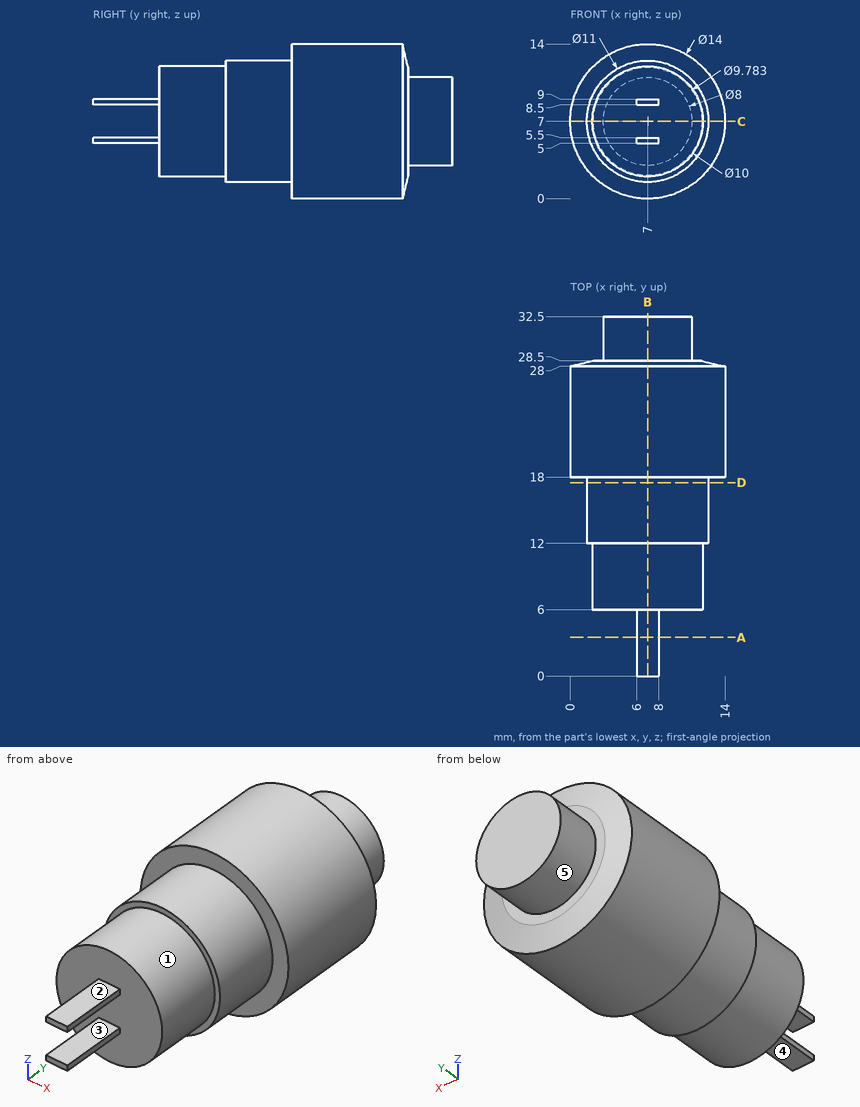
Could you check a few things on this drawing? It's one solid part, dimensions in mm from its lowest x, y, z. A direction names the side the tool comes from. Give positions to 0.01 mm unless a question says otherwise; leave off trailing zeros. Order: outer loops, then holes, each group sorted by start corner. A loop starts at its lowest first (then second) coordinate and runs counter-clockwise, first axis right, second up. Notation, with made-up numbers: (29.25, 40.5) -> (63.25, 40.5) arc R10 cw to (63.25, 52.5) -> close; hole circle Ø2 at (1, 65). An arc over 180 degrees is marked (long way). Use CSV: the item, a comma, the result in double quotes. Start each with the question number.
Item 1: On a 3-axis mill with a long thin cutter (end or side, diameter ignored), from which of +Z, -Z, +X, -X, +Y, -Y can I reach the whole of each face in a straight line? I mean the marked faces 1, 2, 3, 4 and 5. Say none if no direction works.
Item 2: Suppose I cut it at C-C (z = 7). List the corners of the cut face in (x, y) for me, and give its area (3 significant figures).
Item 3: Suppose I cut it at B-B (x = 7). List the corners of the cut face in (y, z) for me.
Item 4: Suppose I cut it at A-A (y = 3.5). List the corners of the cut face in (x, z) for me.
Item 5: I'm going to push flat-ended pins straight in: P1, Ø0.6, axis at y = 4, z = 5, coming from the +X side; P2, Ø1.5, axis at x = 5.5, y = 8, coming from the -Z side; P3, Ø5, axis at x = 4.5, z = 5.5, coming from the -Y side; P4, Ø1, axis at y = 20.5, z = 5, coming from the +X side. Where does each tip first touch, or does it pass through?
Item 6: Suppose I cut it at D-D (y = 17.5). List the corners of the cut face in (x, z) for me.
Item 7: If I drill on probe 1 along Y at (x, z) = (4, 9); probe 2 along Y at (x, z) = (3.5, 9); probe 3 along Z at (x, y) = (5.5, 31), over which ranges is the centre line in solid material (lowest first)? Write a range as [from, to].
Answer block:
1,face 1,"-Y"
1,face 2,"+Z, +X, -X, -Y"
1,face 3,"+X, -X, -Y"
1,face 4,"-Z, +X, -X, -Y"
1,face 5,"+Y"
2,outline,"(0, 18) -> (1.5, 18) -> (1.5, 12) -> (2, 12) -> (2, 6) -> (12, 6) -> (12, 12) -> (12.5, 12) -> (12.5, 18) -> (14, 18) -> (14, 28) -> (11.89, 28.5) -> (11, 28.5) -> (11, 32.5) -> (3, 32.5) -> (3, 28.5) -> (2.11, 28.5) -> (0, 28) -> close"
2,area,"304 mm^2"
3,outline,"(0, 5) -> (6, 5) -> (6, 2) -> (12, 2) -> (12, 1.5) -> (18, 1.5) -> (18, 0) -> (28, 0) -> (28.5, 2.11) -> (28.5, 3) -> (32.5, 3) -> (32.5, 11) -> (28.5, 11) -> (28.5, 11.89) -> (28, 14) -> (18, 14) -> (18, 12.5) -> (12, 12.5) -> (12, 12) -> (6, 12) -> (6, 9) -> (0, 9) -> (0, 8.5) -> (6, 8.5) -> (6, 5.5) -> (0, 5.5) -> close"
4,outline,"(6, 5) -> (8, 5) -> (8, 5.5) -> (6, 5.5) -> close; (6, 8.5) -> (8, 8.5) -> (8, 9) -> (6, 9) -> close"
5,P1,"stops at x = 8"
5,P2,"stops at z = 2.06"
5,P3,"stops at y = 0"
5,P4,"stops at x = 13.84"
6,outline,"circle Ø11 at (7, 7)"
7,probe 1,"y = [6, 32.5]"
7,probe 2,"y = [6, 28.5]"
7,probe 3,"z = [3.29, 10.71]"
